Job drawing, mm, ordinate dimensions from the low corner. One solid piece. A direction names the side the tool comes from. Round coordinates to 2 decimals unless told otherwise and drop trailing zeros. Order: outer loops, then holes, each group sorted by start corner. A loop starts at its lowest first (then second) coordinate and runs counter-clockwise, first axis right, second up. Notation, with made-up numbers: M 43,69.25 L 67,69.25 A12 cw 67,75.25 Z; hole C 89,84.25 d6. An arc over 180 degrees is marked long. Answer as a JSON object with one key per item and string values. Group by question number.
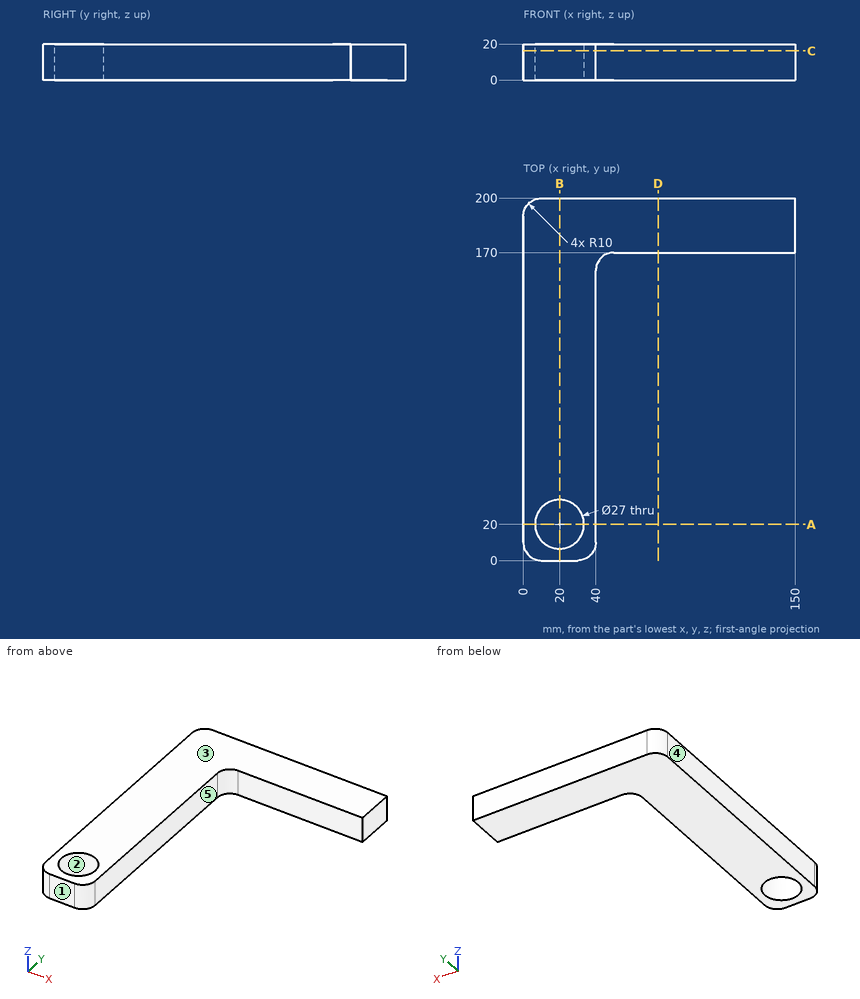
Item 1: Two-plate mould, pull along Y, no slides. Class the marked faces 1, 2 and 3: +Y half, -Y half, draft (parallel to the pull), parting line (faces both ways), or undercut.
Item 2: Drill centre lines: line 1 (Y direction, x = 21, z = 14.75); line 2 (Y direction, x = 31, z = 1.25); line 3 (X direction, y = 65.5, z = 1.25). Where is each one in solid material? Low to high. Write a range as [from, to].
Item 3: 3-axis set-ups, long thin cutter, end or side, ignore diameter. For the marked faces 4 and 5: which of +Z, -Z, +X, -X, +Y, -Y reach the whole face in a straight line?
Item 4: Flat gauge pins, fed straight in: pin 1 Ø6 at (x, z) = (78.5, 8.5) entering from -Y; pin 2 Ø1.5 at (y, z) = (47, 11) entering from +X. Where does each tip first touch, or does it go through?
Item 5: Cut at D-D, the plane x = 74.5. Give the cut face in (y, z).
Item 6: Cut at B-B, the plane x = 20. Give the cut face in (y, z).
Item 7: Cut at A-A, the plane y = 20. Give the cut face in (x, z), and give its area (3 significant figures).
Item 8: Cut at C-C, the plane z = 16.25. Give the cut face in (x, y), and give its area (3 significant figures).
Response values:
{
 "1": {"face 1": "-Y half", "face 2": "undercut", "face 3": "draft"},
 "2": {"line 1": "[0, 6.54], [33.46, 200]", "line 2": "[0.05, 12.17], [27.83, 200]", "line 3": "[0, 40]"},
 "3": {"face 4": "+Z, -Z, -X, +Y, -Y", "face 5": "+Z, -Z, +X, -Y"},
 "4": {"pin 1": "y = 170", "pin 2": "x = 40"},
 "5": {"outline": "M 170,0 L 200,0 L 200,20 L 170,20 Z"},
 "6": {"outline": "M 0,0 L 6.5,0 L 6.5,20 L 0,20 Z; M 33.5,0 L 200,0 L 200,20 L 33.5,20 Z"},
 "7": {"outline": "M 0,0 L 6.5,0 L 6.5,20 L 0,20 Z; M 33.5,0 L 40,0 L 40,20 L 33.5,20 Z", "area": "260 mm^2"},
 "8": {"outline": "M 0,10 A10 ccw 10,0 L 30,0 A10 ccw 40,10 L 40,160 A10 cw 50,170 L 150,170 L 150,200 L 10,200 A10 ccw 0,190 Z; hole C 20,20 d27", "area": "10,700 mm^2"}
}
